Geometry: final body of the model. Coordinates: model frame, mm. Face numbers are marked on the shaded views. Round coordinates to 2 decimals unless told otherwise and drop trailing zeros. Write each loop counter-clockwise with the first axis right and the second up, starting at its lowest first coordinate (ties: lowest second). Pieces come first, ordered by that corner, then holes. Notation, with made-up numbers: M -32,28 L -9,28 A25 ccw -9,65 Z; hole C -13,-6.5 d8. An arc over 180 degrees is marked long. Use one line per item in the form item = value. Start each with the question number.
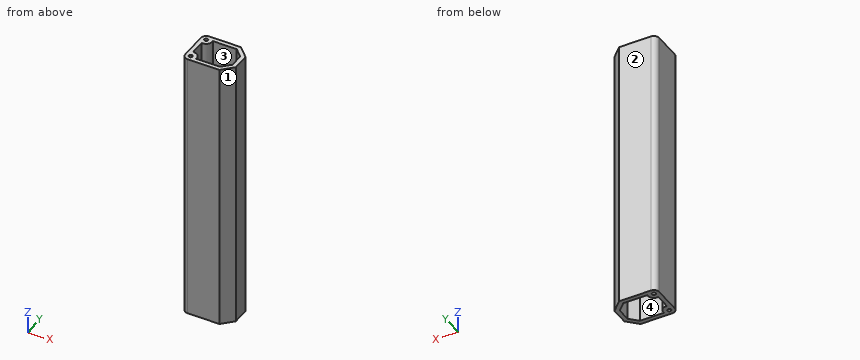
from build123d import *

# Parameters (mm, degrees)
F0_R     = 1.35255
F1_DEPTH = 203.2
F2_T     = -3.175
F3_DEPTH = 3.175
F4_R     = 3.96875


with BuildPart() as f1:
    # F0 (on Top) → F1 (new body)
    with BuildSketch(Plane.XY):
        Polygon((35.120382905, -7.7215365), (27.398846405, 0), (0, 0), (0, -28.143073), (27.398846405, -28.143073), (35.120382905, -20.4215365), align=None)
        with Locations((3.96875, -24.174323)):
            Circle(F0_R, mode=Mode.SUBTRACT)
        with Locations((3.96875, -3.96875)):
            Circle(F0_R, mode=Mode.SUBTRACT)
    extrude(amount=F1_DEPTH)

    # F2
    f2_openings = [f1.faces().sort_by_distance(p)[0] for p in [
        (16.75641, -14.071537, 203.2),
    ]]
    offset(amount=F2_T, openings=f2_openings)

    # F3 (cut, through all): a face of the model
    f3_faces = [f1.faces().sort_by_distance(p)[0] for p in [
        (17.830633935, -14.0715365, 3.175),
    ]]
    extrude(f3_faces, amount=-F3_DEPTH, mode=Mode.SUBTRACT)

    # F4
    f4_edges = [f1.edges().sort_by_distance(p)[0] for p in [
        (0, 0, 101.6),
        (0, -28.143073, 101.6),
    ]]
    fillet(f4_edges, radius=F4_R)


solid = f1.part
1. Section query C-C (x = 13). Return loops of the section in (y, z) (3 decimals).
2. Pull-direction query (X, two-part tool) for the marked faces 1, 2, 3 and 4; classes: released by +X, released by -X, zero draft, split by the parting line, or undercut.
3. Section query A-A (y = -16.5). Return loops of the section in (x, z) (3 decimals), then the cut area to 3 significant figures.
4. Contact query for a flat-ended pin moving along its axis: pin 1 (3 mm diameter, centred on x = 3.5, y = -17, fed in from -Z). Output: stop coordinate, or through.
5. Section query B-B (z = 140). Return loops of the section in (x, y) (1 decimal), then the cut area to 3 significant figures.
6. Ray query, probe 1 along X at (y, z) = (-17.25, 104) (3 decimals); probe 2 along Y at (x, z) = (3, 59.5); probe 3 along Y at (x, z) = (10, 153.5) (3 decimals). Return the intervals inside material, ascending.
Checks:
q1.outline = M -28.143,0 L -24.968,0 L -24.968,203.2 L -28.143,203.2 Z; M -3.175,0 L 0,0 L 0,203.2 L -3.175,203.2 Z
q2.face_1 = released by +X
q2.face_2 = zero draft
q2.face_3 = undercut
q2.face_4 = undercut
q3.outline = M 0,0 L 3.175,0 L 3.175,203.2 L 0,203.2 Z; M 31.945,0 L 35.12,0 L 35.12,203.2 L 31.945,203.2 Z
q3.area = 1,290 mm^2
q4.pin_1 = 0
q5.outline = M 0,-24.2 A4 ccw 4,-28.1 L 27.4,-28.1 L 35.1,-20.4 L 35.1,-7.7 L 27.4,0 L 4,0 A4 ccw 0,-4 Z; hole C 4,-24.2 d2.7; hole C 4,-4 d2.7; hole M 3.2,-19.7 A4.5 cw 8.4,-25 L 26.1,-25 L 31.9,-19.1 L 31.9,-9 L 26.1,-3.2 L 8.4,-3.2 A4.5 cw 3.2,-8.4 Z
q5.area = 366 mm^2
q6.probe_1 = 0 to 3.175, 31.945 to 35.12
q6.probe_2 = -28.02 to -25.12, -23.23 to -4.91, -3.02 to -0.12
q6.probe_3 = -28.143 to -24.968, -3.175 to 0
